Part model, mm, in its own coordinate system. A direction names the side the tool comes from. Give positions to 0.01 mm unless a question says otherwise; leave off trailing zeros.
from build123d import *

# Parameters (mm, degrees)
PAD103_DEPTH            = 4
POCKET044_DEPTH         = 2.75
POCKET045_DEPTH         = 2.5
SKETCH192_R             = 1.5
PAD104_DEPTH            = 6
FILLET006_R             = 3
FILLET007_R             = 1.5
SKETCH221_R             = 1
PAD116_DEPTH            = 6
BODY154_ROLL_ANGLE      = -90
BODY154_PLACEMENT_ANGLE = 2


with BuildPart() as part:
    # Sketch188 → Pad103 (new body, symmetric)
    with BuildSketch(Plane.XZ):
        with BuildLine():
            Line((-22, 0), (-3, 0))
            Line((-3, 0), (-3, -1.5))
            ThreePointArc((-3, -1.5), (0, -4.5), (3, -1.5))
            Line((3, 0), (3, -1.5))
            Line((3, 0), (22, 0))
            Line((22, 0), (28, -2))
            Line((28, -2), (28, 4))
            Line((28, 4), (26, 9))
            ThreePointArc((26, 9), (21.180343, 9.814691), (16.562583, 8.211851))
            ThreePointArc((-16.562583, 8.211851), (0, 3.225464), (16.562583, 8.211851))
            ThreePointArc((-16.562583, 8.211851), (-21.180343, 9.814691), (-26, 9))
            Line((-28, 4), (-26, 9))
            Line((-28, -2), (-28, 4))
            Line((-22, 0), (-28, -2))
        make_face()
    extrude(amount=PAD103_DEPTH, both=True)

    # Sketch190 → Pocket044 (cut, symmetric)
    with BuildSketch(Plane.XZ):
        with BuildLine():
            ThreePointArc((-19, 4), (-15.123106, 2.507577), (-11, 2))
            Line((-11, 0), (-11, 2))
            Line((-11, 0), (-19, 0))
            Line((-19, 0), (-19, 4))
        make_face()
        with BuildLine():
            ThreePointArc((11, 2), (15.123106, 2.507577), (19, 4))
            Line((19, 0), (19, 4))
            Line((11, 0), (19, 0))
            Line((11, 0), (11, 2))
        make_face()
    extrude(amount=POCKET044_DEPTH, both=True, mode=Mode.SUBTRACT)

    # Sketch191 → Pocket045 (cut, symmetric)
    with BuildSketch(Plane.XZ):
        Polygon((-26, -2), (-26, 4), (-24, 7), (-20, 7), (-20, -2), align=None)
        Polygon((-10, -2), (-10, 3), (-4, 2), (-4, -2), align=None)
        Polygon((10, -2), (10, 3), (4, 2), (4, -2), align=None)
        Polygon((26, -2), (26, 4), (24, 7), (20, 7), (20, -2), align=None)
    extrude(amount=POCKET045_DEPTH, both=True, mode=Mode.SUBTRACT)

    # Sketch192 → Pad104 (join, symmetric)
    with BuildSketch(Plane.XZ):
        with Locations((0, -1.5)):
            Circle(SKETCH192_R)
    extrude(amount=PAD104_DEPTH, both=True)

    # Fillet006
    fillet006_edges = [part.edges().sort_by_distance(p)[0] for p in [
        (-28, 0, 4),
        (-26, 0, 9),
        (26, 0, 9),
        (28, 0, 4),
    ]]
    fillet(fillet006_edges, radius=FILLET006_R)

    # Fillet007
    fillet007_edges = [part.edges().sort_by_distance(p)[0] for p in [
        (-28, 4, 0.711126),
        (-27.143844, 4, 6.140391),
        (-25.699112, 4, 8.881973),
        (-20.375073, 4, 9.713888),
        (0, 4, 3.225464),
        (20.375073, 4, 9.713888),
        (25.699112, 4, 8.881973),
        (27.143844, 4, 6.140391),
        (28, 4, 0.711126),
        (-27.945869, 4, 3.989575),
        (27.945869, 4, 3.989575),
        (-28, -4, 0.711126),
        (-27.945869, -4, 3.989575),
        (-27.143844, -4, 6.140391),
        (-25.699112, -4, 8.881973),
        (-20.375073, -4, 9.713888),
        (0, -4, 3.225464),
        (20.375073, -4, 9.713888),
        (25.699112, -4, 8.881973),
        (27.143844, -4, 6.140391),
        (27.945869, -4, 3.989575),
        (28, -4, 0.711126),
    ]]
    fillet(fillet007_edges, radius=FILLET007_R)

    # Sketch221 → Pad116 (join, symmetric)
    with BuildSketch(Plane.XZ):
        with Locations((-26, -0.6)):
            Circle(SKETCH221_R)
        with Locations((26, -0.6)):
            Circle(SKETCH221_R)
    extrude(amount=PAD116_DEPTH, both=True)


with BuildPart() as part_1:
    # Body147 placement: moved
    add(part.part.moved(Location((0, 0, -1))))


with BuildPart() as part_2:
    # Body154 roll: moved
    add(part_1.part.rotate(Axis((0, 0, 0), (1, 0, 0)), BODY154_ROLL_ANGLE))


with BuildPart() as part_3:
    # Body154 placement: moved
    add(part_2.part.moved(Location((-3, 18, 0))).rotate(Axis((-3, 18, 0), (0, 0, 1)), BODY154_PLACEMENT_ANGLE))


solid = part_3.part
1) Drill centre lines: L1, parallel to Z at x = -28, y = 20.5; L2, parallel to X at y = 15, z = 5.5; L3, parallel to X at y = 23.5, z = -1.75. Where is each one in solid material? Low to high.
Check result:
L1: z = -4 to -2.5, 2.5 to 4
L2: x = -29.8 to -28.06, -4.33 to -1.5
L3: x = -29.84 to -17.79, 9.54 to 16.82, 21.73 to 24.21
2) 3-axis set-ups, long thin cutter, end or side, ignore diameter. For faces 4 (the cylindrical face through (-29.896, 22.068, 3.549)), 5 (the cylindrical face through (-3, 17, -5)), 6 (the flat face through (-26.46, 15.67, 3.26)): which of +Z, -Z, +X, -X, +Y, -Y reach the whole face in a straight line?
Check result:
face 4: +Z, -X, +Y
face 5: -Z
face 6: +Z, -Z, -Y
3) Flat gauge pins, fed straight in: P1, Ø4.5, axis at x = 13, y = 19.5, coming from the +Z side; P2, Ø6, axis at x = 4, y = 23.5, coming from the -Z side; P3, Ø5, axis at x = -23, z = -0.5, coming from the +Y side. Where does each tip first touch, or does it go through?
Check result:
P1: stops at z = 4
P2: stops at z = -3.88
P3: stops at y = 26.08
4) Mould opens along Z. For faces 1 (the cylindrical face through (-28.97, 24.97, 0.04)), 2 (the flat face through (-29, 16, 6)), 3 (the flat face through (3.985, 19.752, -0.035)) say: +Z half, -Z half, draft (parallel to the pull), parting line (faces both ways), or undercut.
Check result:
face 1: draft
face 2: +Z half
face 3: undercut
